Geometry check sheet. Reference: the model listing, model coordinates, mm. Face numbers are marked on the shaded views. A direction names the side the tool comes from. Round coordinates to 2 decimals unless told otherwise and drop trailing zeros. Write each loop counter-clockwise with the first axis right and the second up, starting at its lowest first coordinate (ties: lowest second). Pieces come first, ordered by that corner, then holes. Notation, with made-up numbers: (54, 86) -> (79, 86) arc R25 cw to (79, 107) -> close; hole circle Ø1 at (70.5, 14.25). An arc over 180 degrees is marked (long way). Use a Markdown table: item, result.
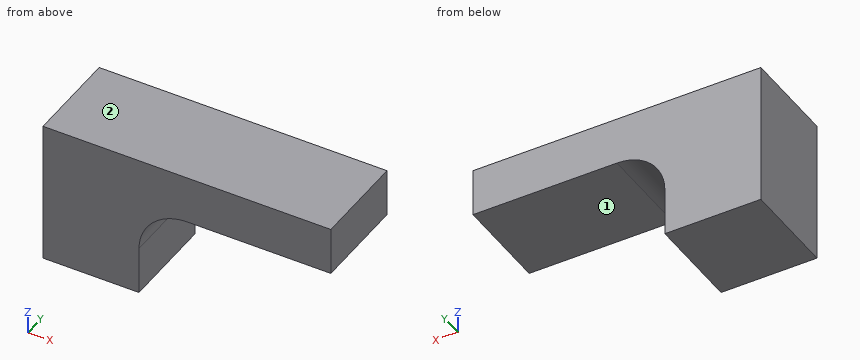
```python
from build123d import *

# Parameters (mm, degrees)
BOSS_EXTRUDE1_DEPTH = 20


with BuildPart() as part:
    # Sketch2 → Boss-Extrude1 (new body)
    with BuildSketch(Plane(origin=(0, 0, 0), x_dir=(1, 0, 0), z_dir=(0, 1, 0))):
        with BuildLine():
            Line((0, 0), (0, -10))
            ThreePointArc((0, -10), (2.928932188, -17.071067812), (10, -20))
            Line((10, -20), (40, -20))
            Line((40, -20), (40, -30))
            Line((40, -30), (-20, -30))
            Line((-20, -30), (-20, 0))
            Line((-20, 0), (0, 0))
        make_face()
    extrude(amount=BOSS_EXTRUDE1_DEPTH)


solid = part.part
```
(1) Section check C-C on z = 6.5. Record the cut outline in (x, y), plus the area to 3 significant figures.
A:
| item | result |
|---|---|
| outline | (-20, 0) -> (0, 0) -> (0, 20) -> (-20, 20) -> close |
| area | 400 mm2 |
(2) Thickness scan on line 1 (X direction, y = 18.75, z = 3.75); line 2 (Z direction, x = 20.5, y = 9.25); line 3 (X direction, y = 7, z = 14.75). Record the ranges inside material, lowest first.
A:
| item | result |
|---|---|
| line 1 | x = -20 to 0 |
| line 2 | z = 20 to 30 |
| line 3 | x = -20 to 1.2 |
(3) Gauge pin test, flat ends, axial feed: pin 1 Ø2 at (x, y) = (20, 2.5) entering from -Z; pin 2 Ø10 at (x, z) = (33, 22.5) entering from -Y; pin 3 Ø8 at (y, z) = (8, 4) entering from +X; pin 4 Ø4 at (y, z) = (8, 9.5) entering from +X. Record the tip position at first contact, or that the pin passes through.
A:
| item | result |
|---|---|
| pin 1 | stops at z = 20 |
| pin 2 | stops at y = 0 |
| pin 3 | stops at x = 0 |
| pin 4 | stops at x = 0.11 |
(4) Section check A-A on y = 8. Record the cut outline in (x, z).
A:
| item | result |
|---|---|
| outline | (-20, 0) -> (0, 0) -> (0, 10) arc R10 cw to (10, 20) -> (40, 20) -> (40, 30) -> (-20, 30) -> close |
(5) Access from +Z, -Z, +X, -X, +Y, -Y to the whole of each face (thin tool, end or side, straight path). Record for the marked faces 1 and 2.
A:
| item | result |
|---|---|
| face 1 | -Z, +X, +Y, -Y |
| face 2 | +Z, +X, -X, +Y, -Y |
(6) Section check B-B on x = 30. Record the cut outline in (y, z), plus the area to 3 significant figures.
A:
| item | result |
|---|---|
| outline | (0, 20) -> (20, 20) -> (20, 30) -> (0, 30) -> close |
| area | 200 mm2 |
